Here's how the part is built. I have some questions about the finished solid (model axes, mm). A direction names the side the tool comes from. Give positions to 0.01 mm unless a question says otherwise; leave off trailing zeros. Order: outer loops, then holes, each group sorted by start corner. A loop starts at its lowest first (then second) coordinate and runs counter-clockwise, first axis right, second up.
from build123d import *

# Parameters (mm, degrees)
CROQUIS1_R                = 2.5
SALIENTE_EXTRUIR1_DEPTH   = 10
CROQUIS2_R                = 1
CORTAR_EXTRUIR1_DEPTH     = 4
SALIENTE_EXTRUIR2_DEPTH   = 13.5
CROQUIS4_R                = 3
CORTAR_EXTRUIR2_DEPTH     = 1
REDONDEO1_R               = 2
CORTAR_EXTRUIR3_START     = -2.598076211
CORTAR_EXTRUIR3_OUTLINE_W = 6
CORTAR_EXTRUIR3_OUTLINE_H = 10
CORTAR_EXTRUIR3_DEPTH     = 2.598076211


# Read off the part's stored shape, not the designer's step: Cortar-Extruir3
with BuildPart() as part:
    # Croquis1 → Saliente-Extruir1 (new body)
    with BuildSketch(Plane.XY):
        with BuildLine():
            Line((-106.231635218, 22.700651543), (-131.231635218, 22.700651543))
            Line((-131.231635218, 22.700651543), (-131.231635218, 20.200651543))
            ThreePointArc((-131.231635218, 20.200651543), (-135.231635218, 16.200651543), (-131.231635218, 12.200651543))
            Line((-131.231635218, 12.200651543), (-125.231635218, 12.200651543))
            Line((-125.231635218, 12.200651543), (-125.231635218, 18.700651543))
            Line((-125.231635218, 18.700651543), (-106.231635218, 18.700651543))
            Line((-106.231635218, 18.700651543), (-106.231635218, 22.700651543))
        make_face()
        with Locations((-131.231635218, 16.200651543)):
            Circle(CROQUIS1_R, mode=Mode.SUBTRACT)
    extrude(amount=SALIENTE_EXTRUIR1_DEPTH)

    # Croquis2 → Cortar-Extruir1 (cut)
    with BuildSketch(Plane.XZ.offset(-18.700651543)):
        with Locations(Location((-119.231635218, 5, 0), (0, 0, 270))):
            Circle(CROQUIS2_R)
        Polygon((-106.231635218, 0), (-106.231635218, 10), (-112.00513791, 0), align=None)
    extrude(amount=-CORTAR_EXTRUIR1_DEPTH, mode=Mode.SUBTRACT)

    # Croquis3 → Saliente-Extruir2 (add)
    with BuildSketch(Plane.XZ.offset(-18.700651543)):
        Polygon((-106.231635218, 10), (-108.231635218, 10), (-114.00513791, 0), (-112.00513791, 0), align=None)
    extrude(amount=-SALIENTE_EXTRUIR2_DEPTH)

    # Croquis4 → Cortar-Extruir2 (cut)
    with BuildSketch(Plane.XZ.offset(-18.700651543)):
        with Locations(Location((-119.231635218, 5, 0), (0, 0, 270))):
            Circle(CROQUIS4_R)
    extrude(amount=-CORTAR_EXTRUIR2_DEPTH, mode=Mode.SUBTRACT)

    # Redondeo1
    redondeo1_edges = [part.edges().sort_by_distance(p)[0] for p in [
        (-125.231635218, 12.200651543, 5),
        (-131.231635218, 22.700651543, 5),
    ]]
    fillet(redondeo1_edges, radius=REDONDEO1_R)

    # Simetría1: part across plane


with BuildPart() as part_1:
    add(part.part)
    add(part.part.mirror(Plane(origin=(0, 32.200651543, 0), x_dir=(0, 0, 1), z_dir=(0, -1, 0))))

    # Cortar-Extruir3 outline → Cortar-Extruir3 (cut)
    with BuildSketch(Plane.XY.offset(10).offset(CORTAR_EXTRUIR3_START)):
        with Locations((-108, 27.700651543)):
            Rectangle(CORTAR_EXTRUIR3_OUTLINE_W, CORTAR_EXTRUIR3_OUTLINE_H)
    extrude(amount=CORTAR_EXTRUIR3_DEPTH, mode=Mode.SUBTRACT)


solid = part_1.part
Q1. For faces 1 (the face through (-116, 45.701, 5)), 2 (the face through (-116, 18.701, 5)), 3 (the face through (-109, 28, 7.402)), 4 (the face through (-121.893, 45.208, 3.616)), which set-ups out of +Z, -Z, +X, -X, +Y, -Y let a thin tool reach every point of the face, with its end or its side?
Filled sheet:
face 1: +Z, -Z, +X, +Y
face 2: +Z, -Z, +X, -Y
face 3: +Z, +X, -X
face 4: +Y
Q2. I need wall thicknesses on L1, parallel to Y at x = -107.25, z = 8.75; L2, parallel to Y at x = -128.5, z = 2.25; L3, parallel to Y at x = -129, z = 8. Which ranges of each line are inside material? Lowest first, please.
Filled sheet:
L1: y = 18.7 to 22.7, 32.7 to 45.7
L2: y = 12.2 to 22.7, 41.7 to 52.2
L3: y = 12.2 to 15.07, 17.33 to 22.7, 41.7 to 47.07, 49.33 to 52.2
Q3. If we section it at B-B on z = 5: Give the number of separate pieces and of enclosed holes in the cut face, plus the area to 3 significant figures.
Filled sheet:
separate pieces: 3
enclosed holes: 2
area: 276 mm2
Q4. If we section it at C-C on y = 42.5: List the corners of the cut face in (x, z) for me, plus the area to 3 significant figures.
Filled sheet:
outline: (-130.83, 0) - (-112.01, 0) - (-106.23, 10) - (-130.83, 10) - close; hole circle Ø2 at (-119.23, 5)
area: 214 mm2
Q5. If we section it at A-A on x = -123.25: List the corners of the cut face in (y, z) for me, plus the area to 3 significant figures.
Filled sheet:
outline: (18.7, 0) - (22.7, 0) - (22.7, 10) - (18.7, 10) - close; (41.7, 0) - (45.7, 0) - (45.7, 10) - (41.7, 10) - close
area: 80.0 mm2
Q6. If we section it at D-D on x = -126.5: List the corners of the cut face in (y, z) for me.
Filled sheet:
outline: (12.34, 0) - (22.7, 0) - (22.7, 10) - (12.34, 10) - close; (41.7, 0) - (52.06, 0) - (52.06, 10) - (41.7, 10) - close
Q7. I'm going to push flat-ended pins straight in: P1, Ø1.8, axis at x = -120, z = 6, coming from the +Y side; P2, Ø6, axis at y = 42.5, z = 2, coming from the -X side; P3, Ø3, axis at x = -119.23, z = 5, coming from the -Y side. Where does each tip first touch, or does it pass through?
Filled sheet:
P1: stops at y = 44.7
P2: stops at x = -134.18
P3: stops at y = 19.7
Q8. Thinking about a two-plate mould opening in X: for faces 5 (the face through (-120, 22.701, 6)), 6 (the face through (-130.63, 42.27, 5.07)), 7 (the face through (-120.208, 43.222, 5.217)), which applies, released by +X, released by -X, zero draft, split by the parting line, or undercut?
Filled sheet:
face 5: zero draft
face 6: released by -X
face 7: undercut
